Here's how the part is built. I have some questions about the finished solid (model axes, mm). Coordinates: 2 decimals unless noted, no trailing zeros. Loops run counter-clockwise (first coordinate to the right, second up) from the corner with the lowest first, then second, coordinate; pieces in that order, holes last. Notation, with made-up numbers: M 89,57.5 L 148,57.5 A10 cw 148,74.5 Z; hole C 37.5,77 d9. An arc over 180 degrees is marked long. Use one line per item in the form item = value. Start each with the question number.
(1) Imagine slicing it at C-C, the plane x = 0. Please give me the cut outline in (y, z).
(2) Imagine slicing it at A-A, the plane x = 15.5. Please give me the cut outline in (y, z), and give its area (3 significant figures).
(3) Imagine slicing it at D-D, the plane z = 28. Please give me the cut outline in (x, y).
(4) Will this pin go through, and if not, where does the flat tip stop? P1, Ø6, axis at x = -13, z = -15.5, coming from the -Y side.
(5) Thinking about a two-plate mould opening in X: for faces 1 (the flat face through (15, 6, 0)), 2 (the flat face through (-35, 3, 0)), 3 (the cylindrical face through (-17, 3, 14.6)), which applies, +X half, -X half, draft (parallel to the pull), parting line (faces both ways), or undercut?
(6) Imagine slicing it at B-B, the plane z = 0. Please give me the cut outline in (x, y), and give its area (3 significant figures).
(7) Please list where these lines run through material, in increasing order: L1, parallel to X at y = 1.35, z = 15.5; L2, parallel to X at y = 3, z = -28; L3, parallel to X at y = 3.7, z = 0.
```python
from build123d import *

# Parameters (mm, degrees)
SKETCH4_W           = 70
SKETCH4_H           = 70
SKETCH4_R           = 12
BOSS_EXTRUDE2_DEPTH = 6
SKETCH5_R           = 1.75
CUT_EXTRUDE1_DEPTH  = 50.859803449
SKETCH6_R           = 2.75
CUT_EXTRUDE2_DEPTH  = 50.859803449


with BuildPart() as part:
    # Sketch4 → Boss-Extrude2 (new body)
    with BuildSketch(Plane(origin=(0, 0, 0), x_dir=(1, 0, 0), z_dir=(0, 1, 0))):
        Rectangle(SKETCH4_W, SKETCH4_H)
        with Locations(Location((0, 0, 0), (0, 0, 270))):
            Circle(SKETCH4_R, mode=Mode.SUBTRACT)
    extrude(amount=BOSS_EXTRUDE2_DEPTH)

    # Sketch5 → Cut-Extrude1 (cut, through all)
    with BuildSketch(Plane(origin=(0, 6, 0), x_dir=(1, 0, 0), z_dir=(0, 1, 0))):
        with Locations(Location((-15.5, 15.5, 0), (0, 0, 270))):
            Circle(SKETCH5_R)
        with Locations(Location((15.5, 15.5, 0), (0, 0, 90))):
            Circle(SKETCH5_R)
        with Locations(Location((15.5, -15.5, 0), (0, 0, 270))):
            Circle(SKETCH5_R)
        with Locations(Location((-15.5, -15.5, 0), (0, 0, 90))):
            Circle(SKETCH5_R)
    extrude(amount=-CUT_EXTRUDE1_DEPTH, mode=Mode.SUBTRACT)

    # Sketch6 → Cut-Extrude2 (cut, through all)
    with BuildSketch(Plane(origin=(0, 6, 0), x_dir=(1, 0, 0), z_dir=(0, 1, 0))):
        with Locations(Location((-28, 28, 0), (0, 0, 270))):
            Circle(SKETCH6_R)
        with Locations(Location((28, 28, 0), (0, 0, 90))):
            Circle(SKETCH6_R)
        with Locations(Location((28, -28, 0), (0, 0, 270))):
            Circle(SKETCH6_R)
        with Locations(Location((-28, -28, 0), (0, 0, 90))):
            Circle(SKETCH6_R)
    extrude(amount=-CUT_EXTRUDE2_DEPTH, mode=Mode.SUBTRACT)


solid = part.part
```
Answer:
q1.outline = M 0,-35 L 6,-35 L 6,-12 L 0,-12 Z; M 0,12 L 6,12 L 6,35 L 0,35 Z
q2.outline = M 0,-35 L 6,-35 L 6,-17.25 L 0,-17.25 Z; M 0,-13.75 L 6,-13.75 L 6,13.75 L 0,13.75 Z; M 0,17.25 L 6,17.25 L 6,35 L 0,35 Z
q2.area = 378 mm²
q3.outline = M -35,0 L -30.75,0 L -30.75,6 L -35,6 Z; M -25.25,0 L 25.25,0 L 25.25,6 L -25.25,6 Z; M 30.75,0 L 35,0 L 35,6 L 30.75,6 Z
q4.P1 = 0
q5.face_1 = draft
q5.face_2 = -X half
q5.face_3 = undercut
q6.outline = M -35,0 L -12,0 L -12,6 L -35,6 Z; M 12,0 L 35,0 L 35,6 L 12,6 Z
q6.area = 276 mm²
q7.L1 = -35 to -17.25, -13.75 to 13.75, 17.25 to 35
q7.L2 = -35 to -30.75, -25.25 to 25.25, 30.75 to 35
q7.L3 = -35 to -12, 12 to 35
